from build123d import *

# Parameters (mm, degrees)
BOSS_EXTRU_1_DEPTH           = 10
ESQUISSE2_R                  = 1.5
ENL_V_MAT_EXTRU_1_DEPTH      = 10
ESQUISSE3_R                  = 2.5
ENL_V_MAT_EXTRU_2_DEPTH      = 3
ENL_V_START                  = -3
ESQUISSE4_R                  = 2.5
ENL_V_MAT_EXTRU_3_DEPTH      = 3
ENL_V_MAT_EXTRU_5_DEPTH      = 50.448460785
ENL_V_MAT_EXTRU_5_DEPTH_BACK = 10


with BuildPart() as part:
    # Esquisse1 → Boss.-Extru.1 (new body)
    with BuildSketch(Plane.XY):
        with BuildLine():
            Line((0, 0), (10, 0))
            add(Edge.make_bspline(
                [(10, 0), (9.921489326, 7.148546847), (10.713934518, 12.333283688), (18.75869357, 21.376035051), (34.363019417, 19.898437833), (40, 17.351511011)],
                knots=[0, 0, 0, 0, 0.337628769, 0.409350915, 1, 1, 1, 1], degree=3))
            Line((40, 17.351511011), (40, 18.993822565))
            add(Edge.make_bspline(
                [(0, 0), (-0.039213766, 11.180464065), (8.69921101, 30.121953716), (34.057263146, 28.337308065), (40, 18.993822565)],
                knots=[0, 0, 0, 0, 0.468371503, 1, 1, 1, 1], degree=3))
        make_face()
    extrude(amount=BOSS_EXTRU_1_DEPTH)

    # Esquisse2 → Enlèv. mat.-Extru.1 (cut)
    with BuildSketch(Plane.XY.offset(10)):
        with Locations((4.95185359, 5)):
            Circle(ESQUISSE2_R)
    extrude(amount=-ENL_V_MAT_EXTRU_1_DEPTH, mode=Mode.SUBTRACT)

    # Esquisse3 → Enlèv. mat.-Extru.2 (cut)
    with BuildSketch(Plane.XY.offset(10)):
        with Locations((4.95185359, 5)):
            Circle(ESQUISSE3_R)
    extrude(amount=-ENL_V_MAT_EXTRU_2_DEPTH, mode=Mode.SUBTRACT)

    # Esquisse4 → Enlèv. mat.-Extru.3 (cut)
    with BuildSketch(Plane(origin=(0, 0, 0), x_dir=(-1, 0, 0), z_dir=(0, 0, -1)).offset(ENL_V_START)):
        with Locations(Location((-4.95185359, 5, 0), (0, 0, 180))):
            Circle(ESQUISSE4_R)
    extrude(amount=ENL_V_MAT_EXTRU_3_DEPTH, mode=Mode.SUBTRACT)

    # Esquisse5 → Enlèv. mat.-Extru.5 (cut, two sides: drawn at the far end of the back side and taken through both)
    with BuildSketch(Plane.XY.offset(10).offset(-ENL_V_MAT_EXTRU_5_DEPTH_BACK)):
        with BuildLine():
            Line((40, 17.351511011), (40, 18.993822565))
            Line((40, 18.993822565), (36.925358186, 18.408031117))
            add(Edge.make_bspline(
                [(36.925358186, 18.408031117), (38.102088932, 18.094984676), (39.146032524, 17.737354573), (40, 17.351511011)],
                knots=[0.91052034, 0.91052034, 0.91052034, 0.91052034, 1, 1, 1, 1], degree=3))
        make_face()
    extrude(amount=ENL_V_MAT_EXTRU_5_DEPTH + ENL_V_MAT_EXTRU_5_DEPTH_BACK, mode=Mode.SUBTRACT)


solid = part.part
CAD build for the part. Positions are in the model's coordinates, mm. A direction names the side the tool comes from. Give positions to 0.01 mm unless a question says otherwise; leave off trailing zeros. Put each result on its own line as item: value.
(1) Drop flat-ended pins along their axis: pin 1 Ø2.5 at (x, y) = (4.95, 5) entering from -Z; pin 2 Ø1 at (y, z) = (24, 2) entering from +X; pin 3 Ø1 at (x, z) = (15.5, 5) entering from -Y; pin 4 Ø1 at (y, z) = (11, 3) entering from +X. Give the stop position or say it passes through.
Working result:
pin 1: through
pin 2: x = 35.78
pin 3: y = 16.82
pin 4: x = 11.27
(2) Pull direction X, two halves, no side cores. Call faces 1 (the flat face through (15.4, 17.4, 0)), 2 (the flat face through (38.484, 18.705, 4.93)), 3 (the flat face through (7, 5, 7)), 4 (the cylindrical face through (3.11, 3.31, 1.52)): released by +X, released by -X, zero draft, split by the parting line, or undercut.
Working result:
face 1: zero draft
face 2: released by +X
face 3: undercut
face 4: undercut
(3) Tool access for faces 5 (the flat face through (7, 5, 3)), 6 (the flat face through (15.4, 17.4, 10)), 7 (the cylindrical face through (3.11, 6.69, 8.52)): list every direction of +Z, -Z, +X, -X, +Y, -Y with a clear straight run to the whole face (end or side of a thin tool).
Working result:
face 5: -Z
face 6: +Z, +X, -X, +Y, -Y
face 7: +Z
(4) Wall check: L1, parallel to X at y = 5, z = 2.3; L2, parallel to X at y = 20, z = 6.25; L3, parallel to Y at x = 28, z = 6.25. Give the ranges that are in metal, low to high.
Working result:
L1: 0.27 to 2.45, 7.45 to 10.1
L2: 6.4 to 39.31
L3: 19.65 to 26.85
